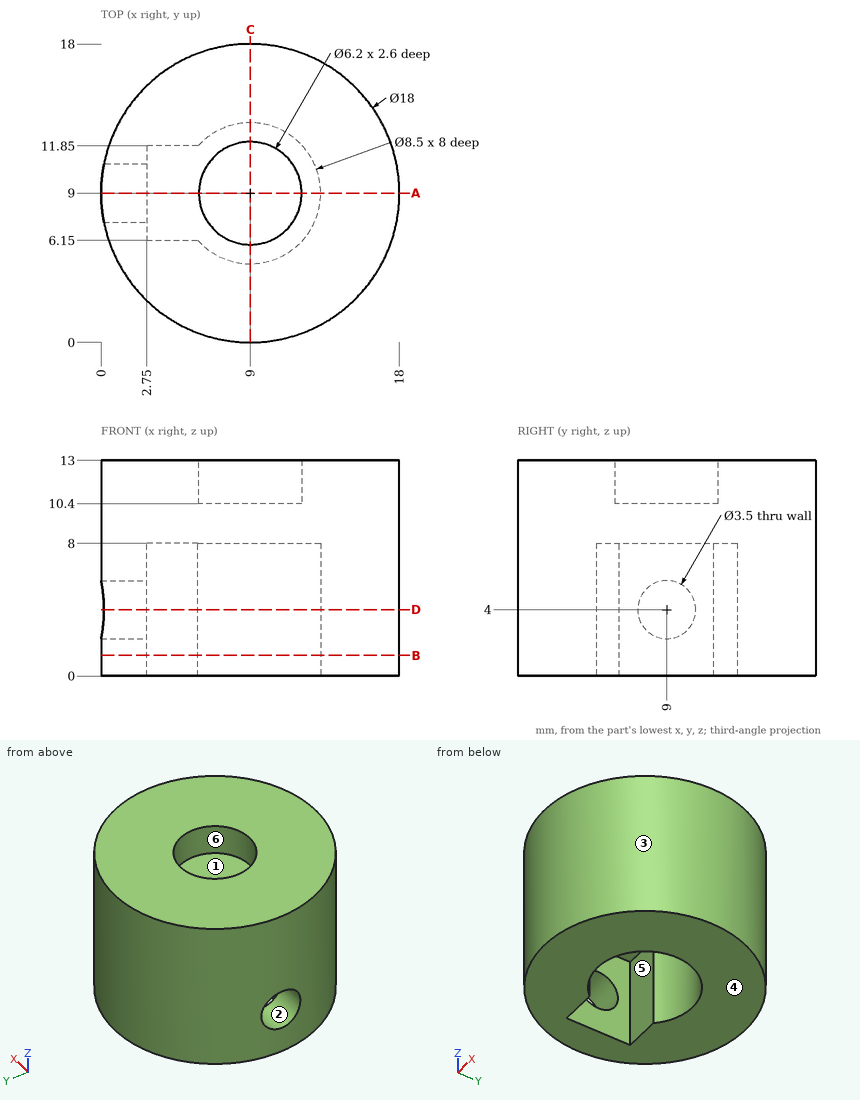
Could you check a few things on this drawing? It's one solid part, dimensions in mm from its lowest x, y, z. A direction names the side the tool comes from. Round coordinates to 2 decimals unless told otherwise and drop trailing zeros. Write each loop counter-clockwise with the first axis right and the second up, starting at its lowest first coordinate (ties: lowest second). Pieces come first, ordered by that corner, then holes.
Q1. If we section it at C-C on x = 9: Write out the boundary of the cut face in (y, z), plus the area to 3 significant figures.
Q2. If we section it at B-B on z = 1.25: Write out the boundary of the cut face in (x, y).
Q3. If we section it at D-D on z = 4: Write out the boundary of the cut face in (x, y), plus the area to 3 significant figures.
Q4. If we section it at A-A on y = 9: Write out the boundary of the cut face in (x, z), plus the area to 3 significant figures.
Q5. Which directions (+Z, -Z, +X, -X, +Y, -Y) give clear straight access to the entire face, cutting with the end or side of a thin tool? Please do the marked faces 4, 5 and 6.
Q6. If we mould it in two halves opening along X, with no side actions, what happens to the marked faces 1, 2 and 3? For each: +X half, -X half, draft (parallel to the pull), parting line (faces both ways), or undercut.
Q7. Please list where these lines run through material, in increasing order: probe 1 along Y at (x, z) = (9, 5.75); probe 2 along Y at (x, z) = (9, 11.95); probe 3 along X at (y, z) = (11, 4).
Q8. Will these pins go through, and if not, where does the flat tip stop? P1, Ø6, axis at y = 14.5, z = 3.5, coming from the -X side; P2, Ø3.5, axis at x = 3.5, z = 5, coming from the +Y side; P3, Ø3.5, axis at x = 4, z = 4.5, coming from the -Y side.
Answer below:
1. outline: (0, 0) - (4.75, 0) - (4.75, 8) - (13.25, 8) - (13.25, 0) - (18, 0) - (18, 13) - (12.1, 13) - (12.1, 10.4) - (5.9, 10.4) - (5.9, 13) - (0, 13) - close
1. area: 150 mm2
2. outline: circle Ø18 at (9, 9); hole (2.75, 6.15) - (5.85, 6.15) arc R4.25 ccw (long way) to (5.85, 11.85) - (2.75, 11.85) - close
3. outline: (0.17, 7.25) arc R9 ccw (long way) to (0.17, 10.75) - (2.75, 10.75) - (2.75, 11.85) - (5.85, 11.85) arc R4.25 cw (long way) to (5.85, 6.15) - (2.75, 6.15) - (2.75, 7.25) - close
3. area: 175 mm2
4. outline: (0, 0) - (2.75, 0) - (2.75, 2.25) - (0, 2.25) - close; (0, 5.75) - (2.75, 5.75) - (2.75, 8) - (13.25, 8) - (13.25, 0) - (18, 0) - (18, 13) - (12.1, 13) - (12.1, 10.4) - (5.9, 10.4) - (5.9, 13) - (0, 13) - close
4. area: 124 mm2
5. face 4: -Z, +X, -X, +Y, -Y
5. face 5: -Z
5. face 6: +Z
6. face 1: undercut
6. face 2: draft
6. face 3: parting line
7. probe 1: y = 0 to 4.75, 13.25 to 18
7. probe 2: y = 0 to 5.9, 12.1 to 18
7. probe 3: x = 0.23 to 2.75, 12.75 to 17.77
8. P1: stops at x = 0.35
8. P2: stops at y = 17.18
8. P3: stops at y = 0.61
